Design review of the part built by this model. Coordinates are the model's own, in mm. A direction names the side the tool comes from. Coordinates: 2 decimals unless noted, no trailing zeros. Write each loop counter-clockwise with the first axis right and the second up, starting at its lowest first coordinate (ties: lowest second). Pieces come first, ordered by that corner, then holes.
Q1. Machinability: for faces 1 (the face through (1.5, -10, 0)), 2 (the face through (-6.5, -15.93, -11.48)), 3 (the face through (-5, -10, -10)), which of the approach directions +Z, -Z, +X, -X, +Y, -Y give a long, thin tool a straight path to every point of the face, cutting with its end or side? Answer none if there is none.
Q2. Add section D-D, the plane x = -0.5. Give the boundary of the cut face in (y, z).
Q3. To check wall thickness, follow probe 1 along Y at (x, z) = (-5, -11.5); probe 2 along Y at (x, z) = (5, -11.6); probe 3 along Z at (x, y) = (-6.5, -2.5). State the ranges of each line that lie inside material, in increasing order.
Q4. Clearance check with flat-ended pins moving along their axes: pin 1 Ø6 at (y, z) = (-10.5, 6.5) entering from +X; pin 2 Ø3 at (x, y) = (-4.5, -13) entering from +Z; pin 3 Ø4 at (y, z) = (-12.5, -7) entering from -X; pin 4 Ø1 at (x, z) = (2.5, 7) entering from +Y. State where each tip first meets the part, or that it passes through.
Q5. The part is to be moulded in two halves that separate along Z. For faces 4 (the face through (0, -10, -13)), 5 (the face through (0.021, -16.033, 1.087)), 6 (the face through (0.021, -4.457, 1.425)), 7 (the face through (-0.6, -20, -6.7)), say which applies: +Z half, -Z half, draft (parallel to the pull), parting line (faces both ways), or undercut.
Q6. Add section A-A, the plane x = 5. Give the boundary of the cut face in (y, z).
Q7. Add section B-B, the plane y = -4. Give the boundary of the cut face in (x, z).
Q8. Add section C-C, the plane z = 2. Give the boundary of the cut face in (x, y), plus the area to 3 significant figures.
from build123d import *

# Parameters (mm, degrees)
F0_W     = 3
F0_H     = 20
F1_DEPTH = 20
F2_R     = 1.5
F3_DEPTH = 9.001
F4_R     = 1.5
F5_DEPTH = 3.001
F6_R     = 1.5
F7_DEPTH = 25
F8_F1_R  = 0.5
F8_F2_R  = 0.5


with BuildPart() as f1:
    # F0 (on Front) → F1 (new body)
    with BuildSketch(Plane.XZ):
        Rectangle(F0_W, F0_H)
        Polygon((7.5, -10), (1.5, -10), (-1.5, -10), (-7.5, -10), (-7.5, -13), (7.5, -13), align=None)
    extrude(amount=F1_DEPTH)

    # F2 (on face) → F3 (cut, through all)
    with BuildSketch(Plane.YZ.offset(1.5)):
        with Locations((-14.8428049088, 2)):
            Circle(F2_R)
        with Locations((-5.8428049088, 2)):
            Circle(F2_R)
    extrude(amount=-F3_DEPTH, mode=Mode.SUBTRACT)

    # F4 (on face) → F5 (cut, through all)
    with BuildSketch(Plane.XY.offset(-10)):
        with Locations((5, -4)):
            Circle(F4_R)
    extrude(amount=-F5_DEPTH, mode=Mode.SUBTRACT)

    # F6 (on face) → F7 (cut)
    with BuildSketch(Plane.XY.offset(-10)):
        with Locations((-5, -16)):
            Circle(F6_R)
    extrude(amount=-F7_DEPTH, mode=Mode.SUBTRACT)

    # F8: fillet of radius 0.5 on 10 edges, made by hand

    # F8_f1
    f8_f1_edges = [f1.edges().sort_by_distance(p)[0] for p in [
        (1.5, -10, -10),
        (-1.5, -10, -10),
    ]]
    fillet(f8_f1_edges, radius=F8_F1_R)

    # F8_f2
    f8_f2_edges = [f1.edges().sort_by_distance(p)[0] for p in [
        (-1.5, -10, 10),
        (1.5, -20, 0.25),
        (-1.5, -20, 0.25),
        (1.5, -10, 10),
        (-1.5, 0, 0.25),
        (1.5, 0, 0.25),
        (0, -20, 10),
        (0, 0, 10),
        (1.6464466094, 0, -9.8535533906),
        (-1.6464466094, 0, -9.8535533906),
        (-1.6464466094, -20, -9.8535533906),
        (1.6464466094, -20, -9.8535533906),
    ]]
    fillet(f8_f2_edges, radius=F8_F2_R)


solid = f1.part
Here are the results:
1. face 1: +Z, +X, +Y, -Y
1. face 2: +Z, -Z
1. face 3: +Z, -X, +Y, -Y
2. outline: (-20, -13) - (0, -13) - (0, 9.5) arc R0.5 ccw to (-0.5, 10) - (-19.5, 10) arc R0.5 ccw to (-20, 9.5) - close; hole circle Ø3 at (-14.84, 2); hole circle Ø3 at (-5.84, 2)
3. probe 1: y = -20 to -17.5, -14.5 to 0
3. probe 2: y = -20 to -5.5, -2.5 to 0
3. probe 3: z = -13 to -10
4. pin 1: stops at x = 1.5
4. pin 2: stops at z = -10
4. pin 3: stops at x = -1.5
4. pin 4: passes through
5. face 4: -Z half
5. face 5: undercut
5. face 6: undercut
5. face 7: draft
6. outline: (-20, -13) - (-5.5, -13) - (-5.5, -10) - (-19.5, -10) arc R0.5 ccw to (-20, -10.5) - close; (-2.5, -13) - (0, -13) - (0, -10.5) arc R0.5 ccw to (-0.5, -10) - (-2.5, -10) - close
7. outline: (-7.5, -13) - (3.5, -13) - (3.5, -10) - (2, -10) arc R0.5 cw to (1.5, -9.5) - (1.5, 9.5) arc R0.5 ccw to (1, 10) - (-1, 10) arc R0.5 ccw to (-1.5, 9.5) - (-1.5, -9.5) arc R0.5 cw to (-2, -10) - (-7.5, -10) - close; (6.5, -13) - (7.5, -13) - (7.5, -10) - (6.5, -10) - close
8. outline: (-1.5, -19.5) arc R0.5 ccw to (-1, -20) - (1, -20) arc R0.5 ccw to (1.5, -19.5) - (1.5, -16.34) - (-1.5, -16.34) - close; (-1.5, -13.34) - (1.5, -13.34) - (1.5, -7.34) - (-1.5, -7.34) - close; (-1.5, -4.34) - (1.5, -4.34) - (1.5, -0.5) arc R0.5 ccw to (1, 0) - (-1, 0) arc R0.5 ccw to (-1.5, -0.5) - close
8. area: 41.8 mm2
